Part model, mm, in its own coordinate system. A direction names the side the tool comes from. Give positions to 0.01 mm unless a question says otherwise; leave off trailing zeros. Order: outer loops, then holes, each group sorted by start corner. A loop starts at its lowest first (then second) coordinate and runs counter-clockwise, first axis right, second up. Notation, with made-up numbers: (86, 19.5) - (140, 19.5) arc R34 cw to (140, 57.5) - close; hole circle Ø11 at (-4, -40). An arc over 180 degrees is marked (long way). Use a Markdown table: item, result. Add a question column.
from build123d import *

# Parameters (mm, degrees)
SKETCH1_W                = 27.5
SKETCH1_H                = 19.5
BOSS_EXTRUDE1_DEPTH      = 2.5
BOSS_EXTRUDE2_DEPTH      = 16.5
BOSS_EXTRUDE2_DEPTH_BACK = 16.5
BOSS_EXTRUDE3_DEPTH      = 21.5
BOSS_EXTRUDE3_DEPTH_BACK = 21.25
CUT_EXTRUDE1_DEPTH       = 37.936693725
SKETCH5_R                = 1.75
CUT_EXTRUDE2_DEPTH       = 37.936693725
CHAMFER1_SIZE            = 5.494954839
CHAMFER1_SIZE_2          = 2
BOSS_EXTRUDE4_REACH      = 31.601
SKETCH6_W                = 6
SKETCH6_H                = 4.75
SKETCH7_W                = 19.5
SKETCH7_H                = 4
CUT_EXTRUDE3_DEPTH       = 2
SKETCH8_W                = 27.5
SKETCH8_H                = 19.5
SKETCH8_W_2              = 24
SKETCH8_H_2              = 13.5
BOSS_EXTRUDE5_DEPTH      = 0.5
FILLET1_R                = 1


with BuildPart() as part:
    # Sketch1 → Boss-Extrude1 (new body)
    with BuildSketch(Plane(origin=(0, 0, 0), x_dir=(1, 0, 0), z_dir=(0, 1, 0))):
        Polygon((-16.5, -14.5), (16.5, -14.5), (20, 12), (21.5, 14.35), (-21.25, 14.35), (-20, 12), align=None)
        Rectangle(SKETCH1_W, SKETCH1_H, mode=Mode.SUBTRACT)
    extrude(amount=BOSS_EXTRUDE1_DEPTH)

    # Sketch2 → Boss-Extrude2 (add, two sides: drawn at the far end of the back side and taken through both)
    with BuildSketch(Plane(origin=(0, 0, 0), x_dir=(0, 0, -1), z_dir=(1, 0, 0)).offset(-BOSS_EXTRUDE2_DEPTH_BACK)):
        Polygon((-14.5, 0), (-16.357862064, -1.672826516), (-17.696123276, -0.186536865), (-14.712421813, 2.5), (-14.5, 2.5), align=None)
    extrude(amount=BOSS_EXTRUDE2_DEPTH + BOSS_EXTRUDE2_DEPTH_BACK)

    # Sketch3 → Boss-Extrude3 (add, two sides: drawn at the far end of the back side and taken through both)
    with BuildSketch(Plane(origin=(0, 0, 0), x_dir=(0, 0, -1), z_dir=(1, 0, 0)).offset(-BOSS_EXTRUDE3_DEPTH_BACK)):
        Polygon((14.35, 2.5), (14.790255348, 2.5), (19.851073289, -3.12060774), (18.364783638, -4.458868953), (14.35, 0), align=None)
    extrude(amount=BOSS_EXTRUDE3_DEPTH + BOSS_EXTRUDE3_DEPTH_BACK)

    # Sketch4 → Cut-Extrude1 (cut, through all)
    with BuildSketch(Plane(origin=(0, 8.473955812, -9.411281375), x_dir=(-1, 0, 0), z_dir=(0, 0.6691306063588619, -0.7431448254773909))):
        Polygon((-20.113700783, -8.038750466), (-16.458708787, 11.769448481), (-23.724996003, 11.769448481), (-23.724996003, -12.049500132), align=None)
        Polygon((20.113700783, -8.038750466), (24.708588094, -12.633637777), (20.852277712, 11.769448481), (16.5, 11.702393792), align=None)
    extrude(amount=-CUT_EXTRUDE1_DEPTH, mode=Mode.SUBTRACT)

    # Sketch5 → Cut-Extrude2 (cut, through all)
    with BuildSketch(Plane(origin=(0, 8.473955812, -9.411281375), x_dir=(-1, 0, 0), z_dir=(0, 0.6691306063588619, -0.7431448254773909))):
        with Locations(Location((-17, -12.352024201, 0), (0, 0, 90))):
            Circle(SKETCH5_R)
        with Locations(Location((17, -12.352024201, 0), (0, 0, 90))):
            Circle(SKETCH5_R)
    extrude(amount=-CUT_EXTRUDE2_DEPTH, mode=Mode.SUBTRACT)

    # Chamfer1
    # the kernel refuses this chamfer: 5.494954839, 2 mm, written as the material it takes off along each edge
    with BuildSketch(Plane(origin=(13.75, 0, 9.75), x_dir=(0, -0.013184058198645777, 0.9999130865277316), z_dir=(-1, 0, 0))) as chamfer1_piece_1_section:
        Polygon((CHAMFER1_SIZE * 0.999913086511, CHAMFER1_SIZE * 0.0131840581984), (-CHAMFER1_SIZE_2 * 0.0131840581986, CHAMFER1_SIZE_2 * 0.999913086528), (0, 0), align=None)
    chamfer1_piece_1 = extrude(amount=27.5, mode=Mode.PRIVATE)
    chamfer1_piece_1 = split(chamfer1_piece_1, bisect_by=Plane(origin=(0, 1.804468024, 12.49593523), z_dir=(0, -0.7431448254773978, -0.6691306063588544)), keep=Keep.TOP, mode=Mode.PRIVATE)
    add(chamfer1_piece_1, mode=Mode.SUBTRACT)

    # Boss-Extrude4: up to this plane
    boss_extrude4_end = Plane(origin=(0, 0, 15.244954839), z_dir=(0, -0.9396926207859098, -0.3420201433256651))
    # Sketch6 → Boss-Extrude4 (add, up to the surface)
    with BuildSketch(Plane.XZ, mode=Mode.PRIVATE) as boss_extrude4_sk1:
        with Locations((-10.75, 12.125)):
            Rectangle(SKETCH6_W, SKETCH6_H)
    boss_extrude4_tool1 = split(extrude(boss_extrude4_sk1.sketch, amount=-BOSS_EXTRUDE4_REACH, mode=Mode.PRIVATE), bisect_by=boss_extrude4_end, keep=Keep.BOTH, mode=Mode.PRIVATE)
    add(boss_extrude4_tool1.solids().sort_by_distance((-10.75, 0, 12.125))[0])
    # Sketch6 → Boss-Extrude4 (add, up to the surface)
    with BuildSketch(Plane.XZ, mode=Mode.PRIVATE) as boss_extrude4_sk2:
        with Locations((10.75, 12.125)):
            Rectangle(SKETCH6_W, SKETCH6_H)
    boss_extrude4_tool2 = split(extrude(boss_extrude4_sk2.sketch, amount=-BOSS_EXTRUDE4_REACH, mode=Mode.PRIVATE), bisect_by=boss_extrude4_end, keep=Keep.BOTH, mode=Mode.PRIVATE)
    add(boss_extrude4_tool2.solids().sort_by_distance((10.75, 0, 12.125))[0])

    # Sketch7 → Cut-Extrude3 (cut)
    with BuildSketch(Plane.XZ):
        with Locations((0, -11.75)):
            Rectangle(SKETCH7_W, SKETCH7_H)
    extrude(amount=-CUT_EXTRUDE3_DEPTH, mode=Mode.SUBTRACT)

    # Sketch8 → Boss-Extrude5 (add)
    with BuildSketch(Plane(origin=(0, 2.5, 0), x_dir=(1, 0, 0), z_dir=(0, 1, 0))):
        Rectangle(SKETCH8_W, SKETCH8_H)
        with Locations((0, 1.75)):
            Rectangle(SKETCH8_W_2, SKETCH8_H_2, mode=Mode.SUBTRACT)
    extrude(amount=-BOSS_EXTRUDE5_DEPTH)

    # Fillet1
    fillet1_edges = [part.edges().sort_by_distance(p)[0] for p in [
        (-0.01445917, 2.5, 14.712421813),
    ]]
    fillet(fillet1_edges, radius=FILLET1_R)


solid = part.part
1. Tool access for faces 5 (the face through (-0.17, -3.78, -19.12)), 6 (the face through (-11, 1, 9.75)): list every direction of +Z, -Z, +X, -X, +Y, -Y with a clear straight run to the whole face (end or side of a thin tool).
2. Mould opens along X. For faces 1 (the face through (12, 1, -9.75)), 2 (the face through (21.5, -2, -17)), 3 (the face through (-0.174, -0.271, -17.285)), 4 (the face through (-21.25, -1, -17)) say: released by +X, released by -X, zero draft, split by the parting line, or undercut.
3. Pin check, flat tips, straight feed: P1, Ø1, axis at x = -12.5, y = 1.5, coming from the +Z side; P2, Ø1.6, axis at y = 1, z = 12, coming from the +X side; P3, Ø2, axis at y = 0, z = 9.5, coming from the +X side. Stop position of each tip, or through.
4. Cut at A-A (x = 1). Write the cut outline in (y, z), plus the area to 3 significant figures.
5. Cut at C-C (x = -11). Write the cut outline in (y, z).
6. Drill centre lines: probe 1 along Y at (x, z) = (-4, -11); probe 2 along X at (y, z) = (0.5, -8); probe 3 along Z at (x, y) = (14, -1.5). Where is each one in solid material? Low to high. Write a range as [from, to].
7. Cut at D-D (z = -9). Write the cut outline in (x, y).
8. Cut at B-B (z = -3). Write the cut outline in (x, y).
Responses:
| question | item | result |
|---|---|---|
| 1 | face 5 | -Z, +X, -X, -Y |
| 1 | face 6 | -Y |
| 2 | face 1 | undercut |
| 2 | face 2 | released by +X |
| 2 | face 3 | zero draft |
| 2 | face 4 | released by -X |
| 3 | P1 | stops at z = 16.38 |
| 3 | P2 | stops at x = 16.94 |
| 3 | P3 | stops at x = 17.29 |
| 4 | outline | (-4.46, -18.36) - (-3.12, -19.85) - (2.5, -14.79) - (2.5, -8.5) - (2, -8.5) - (2, -13.75) - (0, -13.75) - (0, -14.35) - close; (-1.67, 16.36) - (0.46, 13.99) - (2, 9.75) - (2, 5) - (2.5, 5) - (2.5, 14.33) arc R1 ccw to (2.24, 15) - (-0.19, 17.7) - close |
| 4 | area | 33.9 mm² |
| 5 | outline | (-4.46, -18.36) - (-3.12, -19.85) - (2.5, -14.79) - (2.5, -8.5) - (2, -8.5) - (2, -9.75) - (0, -9.75) - (0, -14.35) - close; (-1.67, 16.36) - (0, 14.5) - (0, 9.75) - (2, 9.75) - (2, 5) - (2.5, 5) - (2.5, 14.33) arc R1 ccw to (2.24, 15) - (-0.19, 17.7) - close |
| 6 | probe 1 | y = [2, 2.5] |
| 6 | probe 2 | x = [-19.47, -13.75], [13.75, 19.47] |
| 6 | probe 3 | z = [-18.39, -15.7], [16.17, 16.51] |
| 7 | outline | (-19.6, 0) - (-13.75, 0) - (-13.75, 2) - (13.75, 2) - (13.75, 0) - (19.6, 0) - (19.6, 1.01) - (19.4, 2.5) - (-19.4, 2.5) - (-19.6, 1.03) - close |
| 8 | outline | (-18.81, 0) - (-13.75, 0) - (-13.75, 2) - (-12, 2) - (-12, 2.5) - (-18.67, 2.5) - (-18.81, 1.46) - close; (12, 2) - (13.75, 2) - (13.75, 0) - (18.81, 0) - (18.81, 1.38) - (18.66, 2.5) - (12, 2.5) - close |
